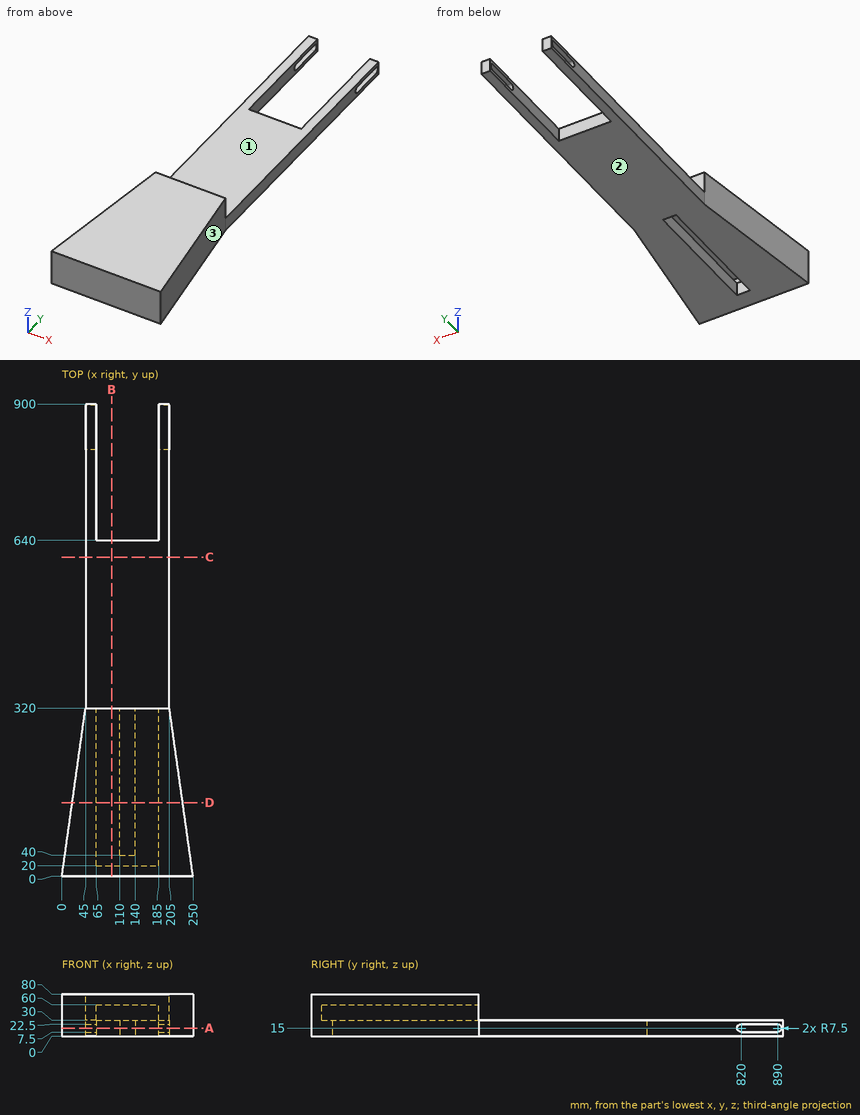
Part print with two shaded views. Sizes in mm from the minimum x, y, z corner. Coordinates: 2 decimals unless noted, no trailing zeros. Loops run counter-clockwise (first coordinate to the right, second up) from the corner with the lowest first, then second, coordinate; pieces in that order, holes last. Notation, with made-up numbers: (9, -30) -> (61, -30) arc R20 ccw to (61, -24) -> close; hole circle Ø7 at (2, 48.25). An arc over 180 degrees is marked (long way). Answer as a JSON object with one key per item and string values.
Q1. Cut at B-B (x = 95). List the corners of the cut face in (y, z).
Report:
{"outline": "(0, 0) -> (640, 0) -> (640, 30) -> (20, 30) -> (20, 60) -> (320, 60) -> (320, 80) -> (0, 80) -> close"}
Q2. Cut at A-A (z = 15). List the corners of the cut face in (x, y), and give its area (3 significant figures).
Report:
{"outline": "(0, 0) -> (250, 0) -> (205, 320) -> (205, 812.5) -> (185, 812.5) -> (185, 640) -> (65, 640) -> (65, 812.5) -> (45, 812.5) -> (45, 320) -> close; (45, 897.5) -> (65, 897.5) -> (65, 900) -> (45, 900) -> close; (185, 897.5) -> (205, 897.5) -> (205, 900) -> (185, 900) -> close; hole (110, 40) -> (140, 40) -> (140, 320) -> (110, 320) -> close", "area": "115,000 mm2"}
Q3. Pull direction Z, two halves, no side cores. Call the marked faces 1, 2 and 3: released by +Z, released by -Z, zero draft, split by the parting line, or undercut.
Report:
{"face 1": "undercut", "face 2": "released by -Z", "face 3": "zero draft"}
Q4. Probe probe 1 along Z at (x, y) = (105.5, 312); probe 2 along Y at (x, z) = (123, 56); probe 3 along X at (y, z) = (659, 10.5). List the from-to ranges inside material, lowest first.
Report:
{"probe 1": "z = 0 to 30, 60 to 80", "probe 2": "y = 0 to 20", "probe 3": "x = 45 to 65, 185 to 205"}
Q5. Cut at C-C (y = 608). List the corners of the cut face in (x, z).
Report:
{"outline": "(45, 0) -> (205, 0) -> (205, 30) -> (45, 30) -> close"}
Q6. Cut at D-D (y = 140). List the corners of the cut face in (x, z), and give its area (4 significant figures).
Report:
{"outline": "(19.69, 0) -> (110, 0) -> (110, 30) -> (65, 30) -> (65, 60) -> (185, 60) -> (185, 30) -> (140, 30) -> (140, 0) -> (230.31, 0) -> (230.31, 80) -> (19.69, 80) -> close", "area": "12,350 mm2"}
Q7. Flat gauge pins, fed straight in: P1, Ø1, axis at x = 135, z = 29, coming from the -Y side; P2, Ø24, axis at y = 764, z = 9, coming from the +X side; P3, Ø10, axis at x = 164, y = 623.5, coming from the +Z side; P4, Ø9, axis at x = 103, z = 48.5, coming from the +Y side. Where does each tip first touch, or does it go through?
Report:
{"P1": "stops at y = 0", "P2": "stops at x = 205", "P3": "stops at z = 30", "P4": "stops at y = 20"}
